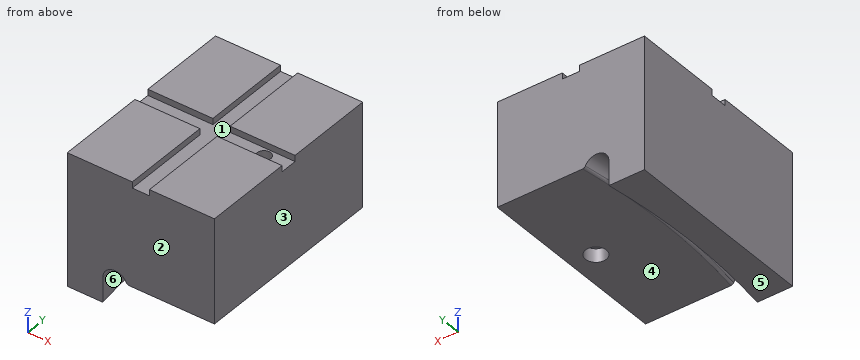
```python
from build123d import *

# Parameters (mm, degrees)
F5_DEPTH  = 108.1010001
F7_DEPTH  = 108.1
F9_DEPTH  = 5
F10_R     = 8.5
F11_DEPTH = 11
F12_R     = 5.5
F13_DEPTH = 69.1


with BuildPart() as f3:
    # F3: sweep along a path in F2
    with BuildLine(Plane.XY.offset(139.4)) as f3_path:
        ThreePointArc((-340.8897771879, 286.0404863105), (-445, 0), (-340.8897771879, -286.0404863105))
    # F0 (on Front) → F3 (sweep)
    with BuildSketch(Plane.XZ):
        with BuildLine():
            Line((-565, 116.4), (-542, 116.4))
            Line((-542, 116.4), (-542, 136.4))
            ThreePointArc((-542, 136.4), (-534.2583426132, 146.1416573868), (-523.0200222717, 140.8))
            ThreePointArc((-523.0200222717, 140.8), (-522.0979034952, 139.7786796564), (-520.7750278397, 139.4))
            Line((-520.7750278397, 139.4), (-445, 139.4))
            Line((-445, 139.4), (-445, 224.5))
            Line((-445, 224.5), (-565, 224.5))
            Line((-565, 224.5), (-565, 116.4))
        make_face()
    sweep(path=f3_path.line)

    # F4 (on face) → F5 (cut, through all)
    with BuildSketch(Plane.XY.offset(224.5)):
        with BuildLine():
            ThreePointArc((-432.8151103622, 363.1749994729), (-515.8719724812, 230.4367765969), (-559.3076076722, 80))
            Line((-559.3076076722, 80), (-445, 80))
            Line((-445, 80), (-445, 0))
            ThreePointArc((-445, 0), (-418.1632162497, 152.1989637799), (-340.8897771879, 286.0404863105))
            Line((-340.8897771879, 286.0404863105), (-432.8151103622, 363.1749994729))
        make_face()
        with BuildLine():
            Line((-445, -80), (-559.3076076722, -80))
            ThreePointArc((-559.3076076722, -80), (-515.8719724812, -230.4367765969), (-432.8151103622, -363.1749994729))
            Line((-432.8151103622, -363.1749994729), (-340.8897771879, -286.0404863105))
            ThreePointArc((-340.8897771879, -286.0404863105), (-418.1632162497, -152.1989637799), (-445, 0))
            Line((-445, 0), (-445, -80))
        make_face()
    extrude(amount=-F5_DEPTH, mode=Mode.SUBTRACT)

    # F6 (on face) → F7 (join, through all)
    with BuildSketch(Plane.XY.offset(224.5)):
        with BuildLine():
            ThreePointArc((-565, 0), (-563.57510517, 40.1011325601), (-559.3076076722, 80))
            Line((-559.3076076722, 80), (-565, 80))
            Line((-565, 80), (-565, 0))
        make_face()
        with BuildLine():
            ThreePointArc((-559.3076076722, -80), (-563.57510517, -40.1011325601), (-565, 0))
            Line((-565, 0), (-565, -80))
            Line((-565, -80), (-559.3076076722, -80))
        make_face()
    extrude(amount=-F7_DEPTH)

    # F8 (on face) → F9 (cut)
    with BuildSketch(Plane.XY.offset(224.5)):
        Polygon((-498, 80), (-512, 80), (-512, 7), (-565, 7), (-565, -7), (-512, -7), (-512, -80), (-498, -80), (-498, -7), (-445, -7), (-445, 7), (-498, 7), align=None)
    extrude(amount=-F9_DEPTH, mode=Mode.SUBTRACT)

    # F10 (on face) → F11 (cut)
    with BuildSketch(Plane(origin=(0, 0, 139.4), x_dir=(1, 0, 0), z_dir=(0, 0, -1))):
        with Locations((-465, 0)):
            Circle(F10_R)
    extrude(amount=-F11_DEPTH, mode=Mode.SUBTRACT)

    # F12 (on face) → F13 (cut, through all)
    with BuildSketch(Plane(origin=(0, 0, 150.4), x_dir=(1, 0, 0), z_dir=(0, 0, -1))):
        with Locations((-465, 0)):
            Circle(F12_R)
    extrude(amount=-F13_DEPTH, mode=Mode.SUBTRACT)


solid = f3.part
```
Geometry: final body of the model. Coordinates: model frame, mm. Face numbers are marked on the shaded views. A direction names the side the tool comes from. Give positions to 0.01 mm unless a question says otherwise; leave off trailing zeros. Order: outer loops, then holes, each group sorted by start corner. A loop starts at its lowest first (then second) coordinate and runs counter-clockwise, first axis right, second up. Notation, with made-up numbers: M -24,-28 L 14,-28 A20 cw 14,-13 Z; hole C -7,-8 d6. An arc over 180 degrees is marked long. Answer as CSV lines item,"result". Start each with the question number.
1) First-contact query: P1, Ø14.5, axis at x = -465, y = 0, coming from the -Z side; P2, Ø4, axis at x = -548, y = 0.5, coming from the +Z side; P3, Ø12, axis at x = -503.5, y = 6, coming from the -Z side. Flat tips, straight axial feed; report the tip coordinate or a pass-through.
2) Mould query, pull axis X, two halves, no side actions, for the marked faces 1, 2 and 3. Classes: +X half, -X half, draft (parallel to the pull), parting line (faces both ways), or undercut.
3) Set-up query: the marked faces 4, 5 and 6. Return all of +Z, -Z, +X, -X, +Y, -Y with unobstructed straight access to the full face (end or side cutting, diameter ignored); none if empty.
4) Cut plane B-B (x = -486). Output: boundary loops of the cut face in (y, z).
5) Cut plane A-A (x = -465). Output: boundary loops of the cut face in (y, z), then the cut area to 3 significant figures.
6) Line query: line 1 (Y direction, x = -465, z = 143); line 2 (X direction, y = 0, z = 198); line 3 (Y direction, x = -465, z = 203.5). Output: solid intervals per line, ascending. Write a range as from..to.
Findings below:
1,P1,"stops at z = 150.4"
1,P2,"stops at z = 219.5"
1,P3,"stops at z = 139.4"
2,face 1,"undercut"
2,face 2,"draft"
2,face 3,"+X half"
3,face 4,"-Z, +X, +Y, -Y"
3,face 5,"-Z, +X, -X, +Y, -Y"
3,face 6,"-Z, +X"
4,outline,"M -80,139.4 L 80,139.4 L 80,224.5 L 7,224.5 L 7,219.5 L -7,219.5 L -7,224.5 L -80,224.5 Z"
5,outline,"M -80,139.4 L -8.5,139.4 L -8.5,150.4 L -5.5,150.4 L -5.5,219.5 L -7,219.5 L -7,224.5 L -80,224.5 Z; M 5.5,150.4 L 8.5,150.4 L 8.5,139.4 L 80,139.4 L 80,224.5 L 7,224.5 L 7,219.5 L 5.5,219.5 Z"
5,area,"12,600 mm²"
6,line 1,"y = -80..-8.5, 8.5..80"
6,line 2,"x = -565..-470.5, -459.5..-445"
6,line 3,"y = -80..-5.5, 5.5..80"
